from build123d import *

# Parameters (mm, degrees)
BOSS_EXTRUDE1_DEPTH = 12
SKETCH5_W           = 3
SKETCH5_H           = 5.5
CUT_EXTRUDE1_DEPTH  = 52


with BuildPart() as part:
    # Sketch4 → Boss-Extrude1 (new body)
    with BuildSketch(Plane(origin=(0, 0, 0), x_dir=(0, 0, -1), z_dir=(1, 0, 0))):
        with BuildLine():
            Line((-13.310160428, -12.59959893), (-13.310160428, -3.59959893))
            ThreePointArc((-13.310160428, -3.59959893), (-12.138587553, -0.771171806), (-9.310160428, 0.40040107))
            Line((-9.310160428, 0.40040107), (7.189839572, 0.40040107))
            ThreePointArc((7.189839572, 0.40040107), (10.018266697, -0.771171806), (11.189839572, -3.59959893))
            Line((11.189839572, -3.59959893), (11.189839572, -12.59959893))
            Line((11.189839572, -12.59959893), (14.189839572, -12.59959893))
            Line((14.189839572, -12.59959893), (14.189839572, -3.59959893))
            ThreePointArc((14.189839572, -3.59959893), (12.13958704, 1.350148538), (7.189839572, 3.40040107))
            Line((7.189839572, 3.40040107), (-9.310160428, 3.40040107))
            ThreePointArc((-9.310160428, 3.40040107), (-14.259907896, 1.350148538), (-16.310160428, -3.59959893))
            Line((-16.310160428, -3.59959893), (-16.310160428, -12.59959893))
            Line((-16.310160428, -12.59959893), (-13.310160428, -12.59959893))
        make_face()
    extrude(amount=BOSS_EXTRUDE1_DEPTH)

    # Sketch5 → Cut-Extrude1 (cut)
    with BuildSketch(Plane.XY.offset(16.310160428)):
        with Locations((1.5, -9.84959893)):
            Rectangle(SKETCH5_W, SKETCH5_H)
        with Locations((10.5, -9.84959893)):
            Rectangle(SKETCH5_W, SKETCH5_H)
    extrude(amount=-CUT_EXTRUDE1_DEPTH, mode=Mode.SUBTRACT)


solid = part.part
Here's how the part is built. I have some questions about the finished solid (model axes, mm). A direction names the side the tool comes from. Give positions to 0.01 mm unless a question says otherwise; leave off trailing zeros. Order: outer loops, then holes, each group sorted by start corner. A loop starts at its lowest first (then second) coordinate and runs counter-clockwise, first axis right, second up. Notation, with made-up numbers: M 56,59.25 L 90,59.25 A33 ccw 90,87.25 Z; hole C 84.5,-12 d5. An arc over 180 degrees is marked long. Answer as a JSON object with one key per item and string values. Group by question number.
1) We'd pull the mould along Z, two halves only. Please class faces 5 (the cylindrical face through (5.916, -0.74, -9.987)), 6 (the flat face through (3, -10, -13)), 7 (the cylindrical face through (5.92, 1.4, 14.21)): pulls with the +Z half, pulls with the -Z half, needs draft (parallel to the pull), parting line crosses it, or undercut.
2) On a 3-axis mill with a long thin cutter (end or side, diameter ignored), from which of +Z, -Z, +X, -X, +Y, -Y can I reach the whole of each face in a straight line? I mean faces 1 (the flat face through (6, 0.4, 1)), 2 (the flat face through (6, -7, 16.31)), 3 (the flat face through (9, -10, 15)), 4 (the flat face through (1, -7.1, 15)). Say none if no direction works.
3) Suppose I cut it at A-A, the plane y = -10.75. Write out the boundary of the cut face in (x, z).
4) Suppose I cut it at B-B, the plane x = 10. Write out the boundary of the cut face in (y, z), plus the area to 3 significant figures.
5) I'm going to push flat-ended pins straight in: pin 1 Ø0.9 at (x, z) = (10, 14.5) entering from -Y; pin 2 Ø8 at (y, z) = (-3, -3.5) entering from -X; pin 3 Ø2.5 at (y, z) = (-11, -13.5) entering from +X; pin 4 Ø4 at (x, z) = (4.5, -3.5) entering from -Y. Where does each tip first touch, or does it pass through?
6) Suppose I cut it at D-D, the plane z = -12. Write out the boundary of the cut face in (x, y), plus the area to 3 significant figures.
7) Suppose I cut it at C-C, the plane y = -6.75. Write out the boundary of the cut face in (x, z).
8) Please list where these lines run through material, in increasing order: L1, parallel to Z at x = 1.5, y = -6.25; L2, parallel to Y at x = 4.25, z = 2.5; L3, parallel to Z at x = 3, y = -2.25. Write a range as [from, to].
Results found:
{
 "1": {"face 5": "undercut", "face 6": "needs draft", "face 7": "pulls with the +Z half"},
 "2": {"face 1": "+X, -X, -Y", "face 2": "+Z, +X, -X, +Y, -Y", "face 3": "+Z, -Z, +X, -Y", "face 4": "+Z, -Z, -X, -Y"},
 "3": {"outline": "M 3,-14.19 L 9,-14.19 L 9,-11.19 L 3,-11.19 Z; M 3,13.31 L 9,13.31 L 9,16.31 L 3,16.31 Z"},
 "4": {"outline": "M -7.1,-14.19 L -3.6,-14.19 A7 ccw 3.4,-7.19 L 3.4,9.31 A7 ccw -3.6,16.31 L -7.1,16.31 L -7.1,13.31 L -3.6,13.31 A4 cw 0.4,9.31 L 0.4,-7.19 A4 cw -3.6,-11.19 L -7.1,-11.19 Z", "area": "122 mm²"},
 "5": {"pin 1": "y = -7.1", "pin 2": "x = 0", "pin 3": "x = 9", "pin 4": "y = 0.4"},
 "6": {"outline": "M 0,-7.1 L 3,-7.1 L 3,-12.6 L 9,-12.6 L 9,-7.1 L 12,-7.1 L 12,1.49 L 0,1.49 Z", "area": "136 mm²"},
 "7": {"outline": "M 0,-14.19 L 12,-14.19 L 12,-11.19 L 0,-11.19 Z; M 0,13.31 L 12,13.31 L 12,16.31 L 0,16.31 Z"},
 "8": {"L1": "[-14.19, -11.19], [13.31, 16.31]", "L2": "[0.4, 3.4]", "L3": "[-14.06, -10.96], [13.08, 16.18]"}
}
